The model under review builds one solid part; all positions refer to its coordinate system, in mm. A direction names the side the tool comes from. Round coordinates to 2 decimals unless told otherwise and drop trailing zeros. Loops run counter-clockwise (first coordinate to the right, second up) from the corner with the lowest first, then second, coordinate; pieces in that order, holes last. Notation, with made-up numbers: M 48,42.25 L 98,42.25 A17 cw 98,59.25 Z; hole C 84.25,28 d9. An arc over 180 degrees is marked long. Answer as a JSON object with one key per item and string values. Group by question number.
Item 1: Tool access review of faces 4 (the face through (0, 2, -6)), 5 (the face through (-2, 2, -25.4)), 6 (the face through (38.1, 2, -32)): name each direction out of +Z, -Z, +X, -X, +Y, -Y from which nothing blocks a thin tool from reaching the whole face with its end or side.
Item 2: Insertion check: P1, Ø2.5, axis at y = 2, z = -34, coming from the -X side; P2, Ø1.4, axis at x = 41.5, y = 1.5, coming from the -Z side; P3, Ø1.4, axis at x = -1, y = 3, coming from the +Z side. Each pin has a flat end and moves straight along its axis. Give the tip position at first contact, or say it passes through.
Item 3: To check wall thickness, follow line 1 (Z direction, x = 19.05, y = 2.05); line 2 (X direction, y = 3.4, z = -19.05); line 3 (X direction, y = 0.5, z = -2). State the ranges of each line that lie inside material, in increasing order.
Item 4: The part is to be moulded in two halves that separate along X. For faces 1 (the face through (19, 4.762, -24)), 2 (the face through (8.586, 2.348, -17.908)), 3 (the face through (-4.762, 2, -19)), say which applies: +X half, -X half, draft (parallel to the pull), parting line (faces both ways), or undercut.
Item 5: Consider section C-C (x = 30). Give the boundary of the cut face in (y, z).
Item 6: Consider section A-A (z = -19.05). Give the boundary of the cut face in (x, y), and give its area (3 significant figures).
Item 7: Consider section D-D (y = 2.3). Give the boundary of the cut face in (x, z).
Item 8: Consider section B-B (x = 19.05). Give the boundary of the cut face in (y, z).
```python
from build123d import *

# Parameters (mm, degrees)
SKETCH1_R           = 1.524
SKETCH1_R_2         = 1.143
BOSS_EXTRUDE1_DEPTH = 4.7625


with BuildPart() as part:
    # Sketch1 → Boss-Extrude1 (new body)
    with BuildSketch(Plane(origin=(0, 0, 0), x_dir=(1, 0, 0), z_dir=(0, 1, 0))):
        Polygon((0, 0), (0, 12.7), (-4.7625, 12.7), (-4.7625, 25.4), (0, 25.4), (0, 38.1), (38.1, 38.1), (38.1, 25.4), (42.8625, 25.4), (42.8625, 12.7), (38.1, 12.7), (38.1, 0), align=None)
        with Locations(Location((19.05, 19.05, 0), (0, 0, 90))):
            Circle(SKETCH1_R, mode=Mode.SUBTRACT)
        with Locations(Location((29.464, 19.05, 0), (0, 0, 90))):
            Circle(SKETCH1_R_2, mode=Mode.SUBTRACT)
        with Locations(Location((19.05, 8.636, 0), (0, 0, 90))):
            Circle(SKETCH1_R_2, mode=Mode.SUBTRACT)
        with Locations(Location((8.636, 19.05, 0), (0, 0, 90))):
            Circle(SKETCH1_R_2, mode=Mode.SUBTRACT)
        with Locations(Location((19.05, 29.464, 0), (0, 0, 90))):
            Circle(SKETCH1_R_2, mode=Mode.SUBTRACT)
    extrude(amount=BOSS_EXTRUDE1_DEPTH)


solid = part.part
```
Geometry results:
{
 "1": {"face 4": "+Z, -X, +Y, -Y", "face 5": "-Z, -X, +Y, -Y", "face 6": "-Z, +X, +Y, -Y"},
 "2": {"P1": "stops at x = 0", "P2": "stops at z = -25.4", "P3": "stops at z = -12.7"},
 "3": {"line 1": "z = -38.1 to -30.61, -28.32 to -20.57, -17.53 to -9.78, -7.49 to 0", "line 2": "x = -4.76 to 7.49, 9.78 to 17.53, 20.57 to 28.32, 30.61 to 42.86", "line 3": "x = 0 to 38.1"},
 "4": {"face 1": "draft", "face 2": "undercut", "face 3": "-X half"},
 "5": {"outline": "M 0,-38.1 L 4.76,-38.1 L 4.76,-20.06 L 0,-20.06 Z; M 0,-18.04 L 4.76,-18.04 L 4.76,0 L 0,0 Z"},
 "6": {"outline": "M -4.76,0 L 7.49,0 L 7.49,4.76 L -4.76,4.76 Z; M 9.78,0 L 17.53,0 L 17.53,4.76 L 9.78,4.76 Z; M 20.57,0 L 28.32,0 L 28.32,4.76 L 20.57,4.76 Z; M 30.61,0 L 42.86,0 L 42.86,4.76 L 30.61,4.76 Z", "area": "191 mm^2"},
 "7": {"outline": "M -4.76,-25.4 L 0,-25.4 L 0,-38.1 L 38.1,-38.1 L 38.1,-25.4 L 42.86,-25.4 L 42.86,-12.7 L 38.1,-12.7 L 38.1,0 L 0,0 L 0,-12.7 L -4.76,-12.7 Z; hole C 8.64,-19.05 d2.29; hole C 19.05,-19.05 d3.05; hole C 19.05,-29.46 d2.29; hole C 19.05,-8.64 d2.29; hole C 29.46,-19.05 d2.29"},
 "8": {"outline": "M 0,-38.1 L 4.76,-38.1 L 4.76,-30.61 L 0,-30.61 Z; M 0,-28.32 L 4.76,-28.32 L 4.76,-20.57 L 0,-20.57 Z; M 0,-17.53 L 4.76,-17.53 L 4.76,-9.78 L 0,-9.78 Z; M 0,-7.49 L 4.76,-7.49 L 4.76,0 L 0,0 Z"}
}
